Geometry: see drawing. Coordinates: mm, zero at the bounding-box minimum. Round coordinates to 2 decimals unless told otherwise and drop trailing zeros. Write each loop counter-clockwise with the first axis right and the second up, starting at its lowest first coordinate (ties: lowest second). Pieces come first, ordered by that corner, then holes. Notation, with made-up numbers: (77, 2) -> (132, 2) arc R23 ccw to (132, 40) -> close; hole circle Ø3 at (-8.75, -20.75). An arc over 180 degrees is marked (long way). Write item = value, one per line.
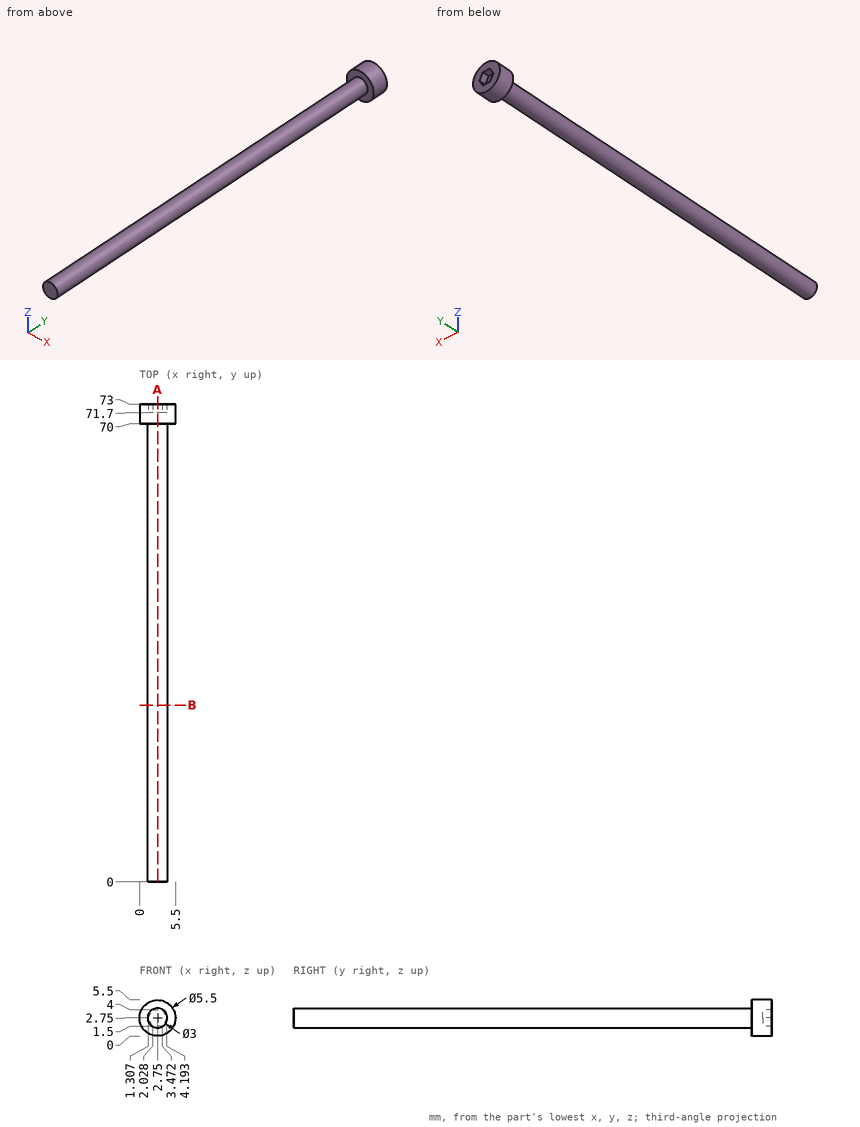
1) Cut plane A-A (x = 2.75). Return the cut outline in (y, z).
Solutions:
outline = (0, 1.25) -> (70, 1.25) -> (70, 0) -> (73, 0) -> (73, 1.5) -> (71.7, 1.5) -> (71.7, 4) -> (73, 4) -> (73, 5.5) -> (70, 5.5) -> (70, 4.25) -> (0, 4.25) -> close
2) First-contact query: P1, Ø1, axis at x = 2.5, y = 42, coming from the -Z side. Flat tip, straight axial feed; report the tip coordinate or a pass-through.
Solutions:
P1 = 1.25
3) Line query: L1, parallel to Y at x = 5.2, z = 3.9; L2, parallel to Y at x = 3.3, z = 2.35; L3, parallel to Z at x = 2.9, y = 29.5. Output: solid intervals per line, ascending. Write a range as from..to.
Solutions:
L1 = 70..73
L2 = 0..71.7
L3 = 1.26..4.24
4) Cut plane B-B (y = 27). Return the cut outline in (x, z).
Solutions:
outline = circle Ø3 at (2.75, 2.75)
